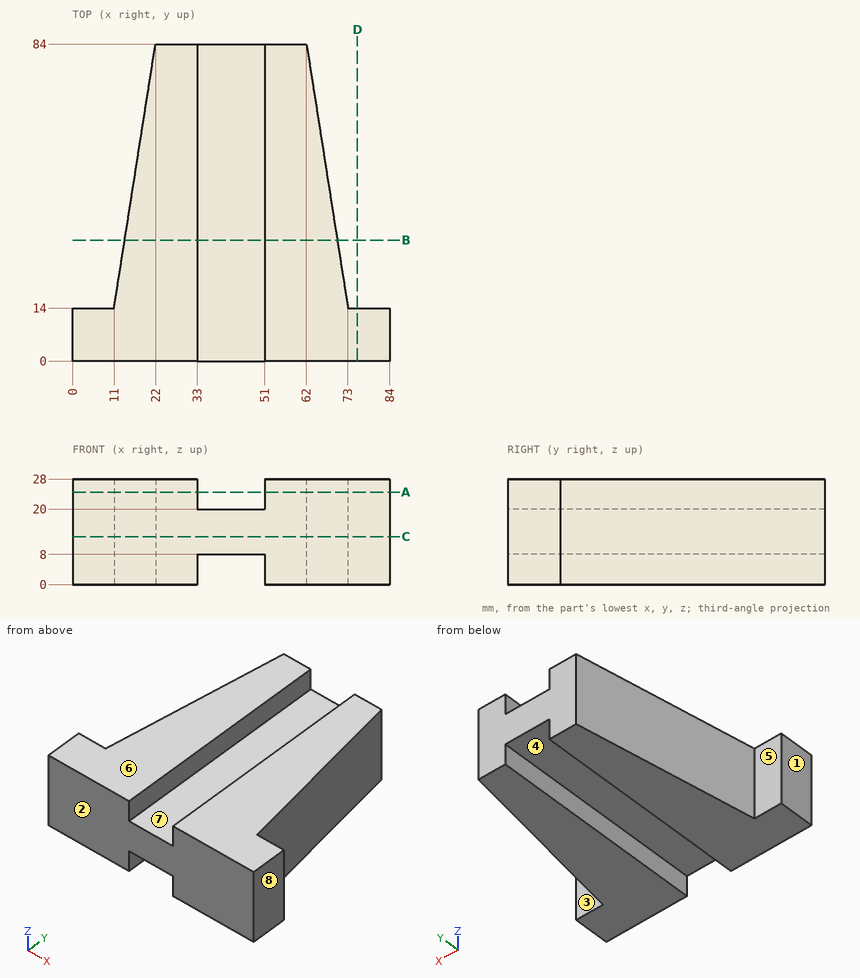
Design review of the part shown in the three views and the two pictorial views. Dimensions are in mm from the part's minimum x, y and z. A direction names the side the tool comes from. Coordinates: 2 decimals unless noted, no trailing zeros. Write each loop counter-clockwise with the first axis right and the second up, starting at its lowest first coordinate (ties: lowest second). Pieces come first, ordered by that corner, then holes. Notation, with made-up numbers: (10, 66) -> (50, 66) arc R18 cw to (50, 89) -> close; hole circle Ø11 at (-21, 6.25). An arc over 180 degrees is marked (long way). Answer in a Markdown table with one row per item.
1. We need section A-A, the plane z = 24.5. State the section outline as (x, y) points, and give its area (3 significant figures).
Answers below:
| item | result |
|---|---|
| outline | (0, 0) -> (33, 0) -> (33, 84) -> (22, 84) -> (11, 14) -> (0, 14) -> close; (51, 0) -> (84, 0) -> (84, 14) -> (73, 14) -> (62, 84) -> (51, 84) -> close |
| area | 3,230 mm^2 |
2. Draft analysis for pull direction X (two halves, no side actions). For the marked faces 6, 7 and 8, state which applies: +X half, -X half, draft (parallel to the pull), parting line (faces both ways), or undercut.
Answers below:
| item | result |
|---|---|
| face 6 | draft |
| face 7 | undercut |
| face 8 | +X half |
3. Wall thickness on probe 1 along X at (y, z) = (7, 5.25); probe 2 along Z at (x, y) = (35, 49.5); probe 3 along X at (y, z) = (18.5, 21.25): over which ranges is each line inside the solid? List them lowest first. Write a range as [from, to].
Answers below:
| item | result |
|---|---|
| probe 1 | x = [0, 33], [51, 84] |
| probe 2 | z = [8, 20] |
| probe 3 | x = [11.71, 33], [51, 72.29] |
4. For the marked faces 1, 2, 3, 4 and 5, list the 3-axis set-ups (+Z, -Z, +X, -X, +Y, -Y) from which the entire face can be reached by the end or side of a thin tool; tool diameter is ignored.
Answers below:
| item | result |
|---|---|
| face 1 | +Z, -Z, -X, +Y, -Y |
| face 2 | +Z, -Z, +X, -X, -Y |
| face 3 | +Z, -Z, +X, +Y |
| face 4 | -Z, +Y, -Y |
| face 5 | +Z, -Z, -X, +Y |
5. We need section D-D, the plane x = 75.5. State the section outline as (y, z) points, and give its area (3 significant figures).
Answers below:
| item | result |
|---|---|
| outline | (0, 0) -> (14, 0) -> (14, 28) -> (0, 28) -> close |
| area | 392 mm^2 |
6. We need section B-B, the plane y = 32. State the section outline as (x, z) points, and give its area (3 significant figures).
Answers below:
| item | result |
|---|---|
| outline | (13.83, 0) -> (33, 0) -> (33, 8) -> (51, 8) -> (51, 0) -> (70.17, 0) -> (70.17, 28) -> (51, 28) -> (51, 20) -> (33, 20) -> (33, 28) -> (13.83, 28) -> close |
| area | 1,290 mm^2 |
7. Clearance check with flat-ended pins moving along their axes: pin 1 Ø14.5 at (x, y) = (44, 38.5) entering from -Z; pin 2 Ø12 at (y, z) = (62, 6) entering from +X; pin 3 Ø6.5 at (y, z) = (44.5, 5.5) entering from -X; pin 4 Ø5.5 at (x, z) = (77.5, 7) entering from +Y. State where each tip first meets the part, or that it passes through.
Answers below:
| item | result |
|---|---|
| pin 1 | stops at z = 0 |
| pin 2 | stops at x = 66.4 |
| pin 3 | stops at x = 15.28 |
| pin 4 | stops at y = 14 |
8. We need section C-C, the plane z = 12.75. State the section outline as (x, y) points.
Answers below:
| item | result |
|---|---|
| outline | (0, 0) -> (84, 0) -> (84, 14) -> (73, 14) -> (62, 84) -> (22, 84) -> (11, 14) -> (0, 14) -> close |
